For this review, use the dimensioned drawing (mm, ordinates from the lowest corner) and the shaded views. A direction names the side the tool comes from. Give positions to 0.01 mm unless a question says otherwise; leave off trailing zeros. Write each loop counter-clockwise with the first axis right and the second up, starting at its lowest first coordinate (ties: lowest second). Pieces come first, ordered by that corner, then holes. Notation, with made-up numbers: M 67.25,-4 L 110.25,-4 A31 ccw 110.25,32 Z; hole C -14.5,-33 d3. An arc over 180 degrees is marked long. Answer in a Markdown table with one row per item.
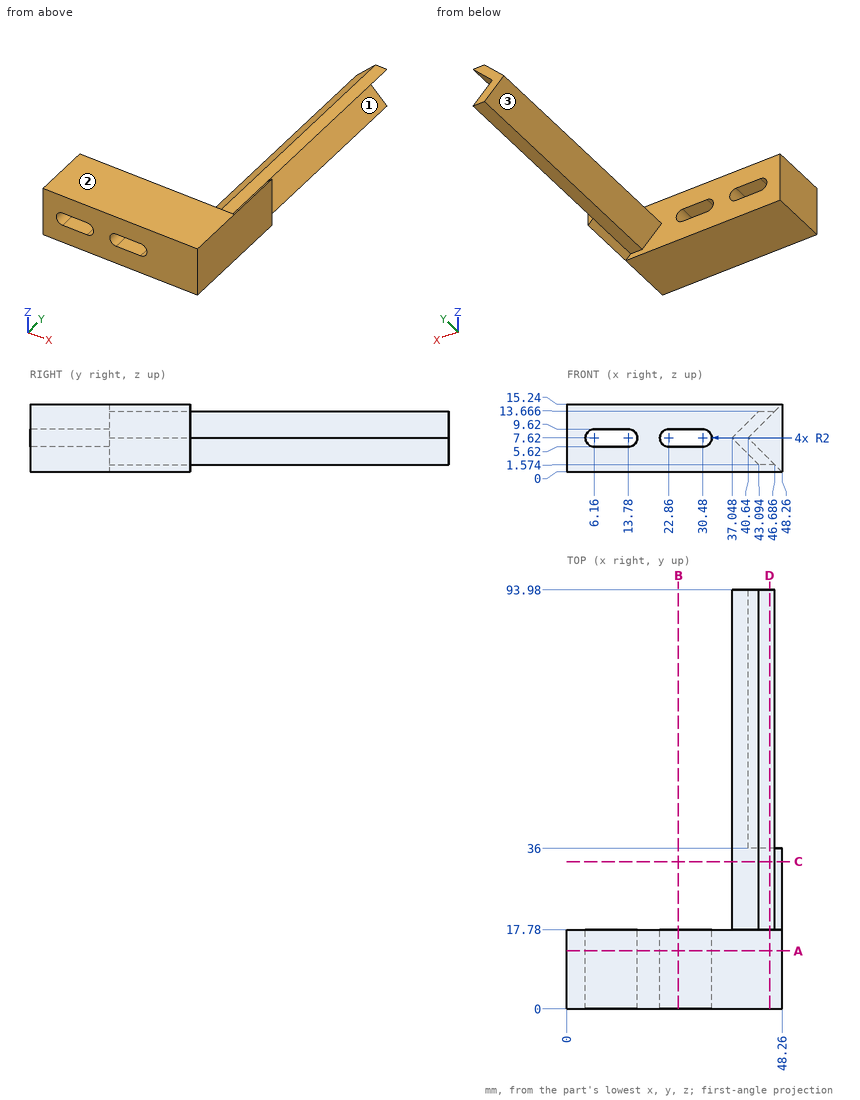
1) Add section A-A (y = 13). Write out the cut boundary in (x, z).
Geometry says:
| item | result |
|---|---|
| outline | M 0,0 L 48.26,0 L 48.26,15.24 L 0,15.24 Z; hole M 6.16,5.62 L 13.78,5.62 A2 ccw 13.78,9.62 L 6.16,9.62 A2 ccw Z; hole M 22.86,5.62 L 30.48,5.62 A2 ccw 30.48,9.62 L 22.86,9.62 A2 ccw Z |
2) Insertion check: P1, Ø1.5, axis at x = 5.5, z = 12, coming from the +Y side; P2, Ø3, axis at y = 78, z = 12, coming from the -X side; P3, Ø4, axis at x = 45, y = 68, coming from the -Z side. Each pin has a flat end and moves straight along its axis. Give the tip position at first contact, or say it passes through.
Geometry says:
| item | result |
|---|---|
| P1 | y = 17.78 |
| P2 | x = 39.93 |
| P3 | z = 1.57 |
3) Add section C-C (y = 33). Write out the cut boundary in (x, z), and give its area (4 significant figures).
Geometry says:
| item | result |
|---|---|
| outline | M 37.05,7.62 L 43.09,1.57 L 46.69,1.57 L 48.26,0 L 48.26,15.24 L 46.69,13.67 L 43.09,13.67 Z |
| area | 101.5 mm^2 |
4) To check wall thickness, follow probe 1 along Y at (x, z) = (17, 4.5); probe 2 along Z at (x, y) = (46, 35.5); probe 3 along X at (y, z) = (82, 5.5). State the ranges of each line that lie inside material, in increasing order. Write a range as [from, to].
Geometry says:
| item | result |
|---|---|
| probe 1 | [0, 17.78] |
| probe 2 | [1.57, 13.67] |
| probe 3 | [39.17, 42.76] |
5) Add section B-B (x = 25). Write out the cut boundary in (y, z), and give its area (3 significant figures).
Geometry says:
| item | result |
|---|---|
| outline | M 0,0 L 17.78,0 L 17.78,5.62 L 0,5.62 Z; M 0,9.62 L 17.78,9.62 L 17.78,15.24 L 0,15.24 Z |
| area | 200 mm^2 |
6) Add section D-D (x = 45.5). Write out the cut boundary in (y, z), and give its area (3 significant figures).
Geometry says:
| item | result |
|---|---|
| outline | M 0,0 L 17.78,0 L 17.78,1.57 L 93.98,1.57 L 93.98,2.76 L 36,2.76 L 36,12.48 L 93.98,12.48 L 93.98,13.67 L 17.78,13.67 L 17.78,15.24 L 0,15.24 Z |
| area | 629 mm^2 |
7) For the marked faces 1, 2 and 3, list the 3-axis set-ups (+Z, -Z, +X, -X, +Y, -Y) from which the entire face can be reached by the end or side of a thin tool; tool diameter is ignored.
Geometry says:
| item | result |
|---|---|
| face 1 | +X, +Y |
| face 2 | +Z, +X, -X, +Y, -Y |
| face 3 | -Z, -X, +Y |
